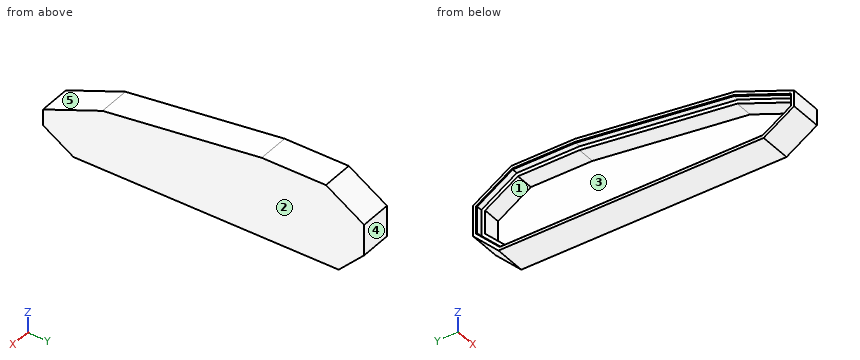
from build123d import *

# Parameters (mm, degrees)
PAD002_DEPTH    = 25.4
THICKNESS001_T  = -6
POCKET_DEPTH    = 5.05
CHAMFER001_SIZE = 0.5


with BuildPart() as part:
    # Sketch002 → Pad002 (new body)
    with BuildSketch(Plane.YZ):
        Polygon((-229.898747, 0), (-20.104522, 0), (0, 20.104522), (0, 44.580842), (-30.23, 63.5), (-81.03, 63.5), (-206.943497, 46.923174), (-254, 27.78354), (-254, 15.08354), align=None)
    extrude(amount=PAD002_DEPTH)

    # Thickness001
    thickness001_openings = [part.faces().sort_by_distance(p)[0] for p in [
        (0, -116.810873, 28.186462),
    ]]
    offset(amount=THICKNESS001_T, openings=thickness001_openings, kind=Kind.INTERSECTION)

    # Sketch003 (on Face11 of Thickness001) → Pocket (cut)
    with BuildSketch(Plane.YZ):
        Polygon((-251.05, 25.798733), (-206.182908, 44.047852), (-80.836647, 60.55), (-31.077013, 60.55), (-2.95, 42.946976), (-2.95, 21.326452), (-21.326452, 2.95), (-229.051734, 2.95), (-251.05, 16.717406), align=None)
        Polygon((-80.636739, 57.5), (-31.952739, 57.5), (-6, 41.257725), (-6, 22.589803), (-22.589803, 6), (-228.176008, 6), (-248, 18.406657), (-248, 23.746644), (-205.396535, 41.075061), align=None, mode=Mode.SUBTRACT)
    extrude(amount=POCKET_DEPTH, mode=Mode.SUBTRACT)

    # Chamfer001
    chamfer001_edges = [part.edges().sort_by_distance(p)[0] for p in [
        (0, -17.013507, 51.748488),
        (0, -55.95683, 60.55),
        (0, -143.509777, 52.298926),
        (0, -228.616454, 34.923292),
        (0, -251.05, 21.25807),
        (0, -240.050867, 9.833703),
        (0, -125.189093, 2.95),
        (0, -12.138226, 12.138226),
        (0, -2.95, 32.136714),
    ]]
    chamfer(chamfer001_edges, length=CHAMFER001_SIZE)


solid = part.part
The model under review builds one solid part; all positions refer to its coordinate system, in mm. Face numbers are marked on the shaded views. A direction names the side the tool comes from. Round coordinates to 2 decimals unless told otherwise and drop trailing zeros. Loops run counter-clockwise (first coordinate to the right, second up) from the corner with the lowest first, then second, coordinate; pieces in that order, holes last. Notation, with made-up numbers: (85.25, 40) -> (141.25, 40) arc R14 ccw to (141.25, 46) -> close; hole circle Ø8 at (29, -12.75). An arc over 180 degrees is marked (long way). One line per question, with ' | ' between items. Start each with the question number.
Item 1: Wall thickness on line 1 along Z through (x, y) = (7.5, -38.5); line 2 along X through (y, z) = (-122.5, 18.5); line 3 along X through (y, z) = (-57, 4): over which ranges is each line inside the solid? List them lowest first. Write a range as [from, to].
Item 2: Add section A-A, the plane x = 12.25. Write out the cut boundary in (y, z), then the cut area to 3 significant figures.
Item 3: Add section C-C, the plane y = -167.5. Write out the cut boundary in (x, z), then the cut area to 3 significant figures.
Item 4: For pin 1 (7 mm diameter, centred on x = 12, y = -144.5, fed in from +Z); pin 2 (2 mm diameter, centred on y = -79.5, z = 57, fed in from -X); pin 3 (12 mm diameter, centred on x = 8, y = -187.5, fed in from +Z), all flat-tipped, find the tip position at first contact; note any pin that passes through.
Item 5: Draft analysis for pull direction Z (two halves, no side actions). For the marked faces 3, 4 and 5, state which applies: +Z half, -Z half, draft (parallel to the pull), parting line (faces both ways), or undercut.
Item 6: Add section B-B, the plane y = -47.5. Write out the cut boundary in (x, z).
Item 7: Machinability: for the marked faces 1 and 2, which of the approach directions +Z, -Z, +X, -X, +Y, -Y give a long, thin tool a straight path to every point of the face, cutting with its end or side? Answer none if there is none.
Return value:
1) line 1: z = [0, 6], [57.5, 63.5] | line 2: x = [19.4, 25.4] | line 3: x = [5.05, 25.4]
2) outline: (-254, 15.08) -> (-229.9, 0) -> (-20.1, 0) -> (0, 20.1) -> (0, 44.58) -> (-30.23, 63.5) -> (-81.03, 63.5) -> (-206.94, 46.92) -> (-254, 27.78) -> close; hole (-248, 18.41) -> (-228.18, 6) -> (-22.59, 6) -> (-6, 22.59) -> (-6, 41.26) -> (-31.95, 57.5) -> (-80.64, 57.5) -> (-205.4, 41.08) -> (-248, 23.75) -> close | area: 3,290 mm2
3) outline: (0, 0) -> (25.4, 0) -> (25.4, 52.12) -> (0, 52.12) -> (0, 49.64) -> (0.5, 49.14) -> (5.05, 49.14) -> (5.05, 46.06) -> (19.4, 46.06) -> (19.4, 6) -> (5.05, 6) -> (5.05, 2.95) -> (0.5, 2.95) -> (0, 2.45) -> close | area: 515 mm2
4) pin 1: stops at z = 55.6 | pin 2: stops at x = 5.05 | pin 3: stops at z = 50.27
5) face 3: undercut | face 4: draft | face 5: +Z half
6) outline: (0, 0) -> (25.4, 0) -> (25.4, 63.5) -> (0, 63.5) -> (0, 61.05) -> (0.5, 60.55) -> (5.05, 60.55) -> (5.05, 57.5) -> (19.4, 57.5) -> (19.4, 6) -> (5.05, 6) -> (5.05, 2.95) -> (0.5, 2.95) -> (0, 2.45) -> close
7) face 1: -X | face 2: +Z, -Z, +X, +Y, -Y
